Can you work these out from the model? Positions are in its coordinate system, mm. A direction names the side the tool comes from. Give positions to 0.01 mm unless a question says otherwise; leave off trailing zeros. Order: outer loops, then holes, each group sorted by start corner. A loop starts at its lowest first (then second) coordinate and runs counter-clockwise, first axis right, second up. Notation, with made-up numbers: (-36, 84) - (15, 84) arc R31 cw to (15, 118) - close; hole circle Ø8 at (-7.75, 62.25). An arc over 180 degrees is marked (long way). One line per question, with ' | ' between items.
```python
from build123d import *

# Parameters (mm, degrees)
ESQUISSE1_W             = 28.5
ESQUISSE1_H             = 46.6
BOSS_EXTRU_1_DEPTH      = 34
ESQUISSE2_R             = 10.15
BOSS_EXTRU_2_DEPTH      = 2
ESQUISSE3_R             = 1
ENL_V_MAT_EXTRU_1_DEPTH = 2


with BuildPart() as part:
    # Esquisse1 → Boss.-Extru.1 (new body)
    with BuildSketch(Plane.XY):
        Rectangle(ESQUISSE1_W, ESQUISSE1_H)
    extrude(amount=BOSS_EXTRU_1_DEPTH)

    # Esquisse2 → Boss.-Extru.2 (add)
    with BuildSketch(Plane.XY.offset(34)):
        with Locations((0, 12)):
            Circle(ESQUISSE2_R)
    extrude(amount=BOSS_EXTRU_2_DEPTH)

    # Esquisse3 → Enlèv. mat.-Extru.1 (cut)
    with BuildSketch(Plane(origin=(0, 23.3, 0), x_dir=(1, 0, 0), z_dir=(0, 1, 0))):
        with Locations(Location((-8.25, -25.319390083, 0), (0, 0, 270))):
            Circle(ESQUISSE3_R)
        with Locations(Location((8.25, -25.319390083, 0), (0, 0, 270))):
            Circle(ESQUISSE3_R)
    extrude(amount=-ENL_V_MAT_EXTRU_1_DEPTH, mode=Mode.SUBTRACT)


solid = part.part
```
(1) If I drill on line 1 (Z direction, x = -3, y = -17.5), over which ranges is the centre line in solid material (lowest first)?
Answer below:
line 1: 0 to 34
(2) On a 3-axis mill with a long thin cutter (end or side, diameter ignored), from which of +Z, -Z, +X, -X, +Y, -Y can I reach the whole of each face in a straight line? I mean faces 1 (the face through (8, 21.3, 25)), 2 (the face through (0, 0, 0)). Say none if no direction works.
Answer below:
face 1: +Y | face 2: -Z, +X, -X, +Y, -Y
(3) If we mould it in two halves opening along X, with no side actions, what happens to faces 3 (the face through (0, -5, 34)), 4 (the face through (-1.321, 22.064, 34.986)), 5 (the face through (14.25, 0, 17)), 6 (the face through (-7.574, 22.314, 24.582))? For each: released by +X, released by -X, zero draft, split by the parting line, or undercut.
Answer below:
face 3: zero draft | face 4: split by the parting line | face 5: released by +X | face 6: undercut
(4) Imagine slicing it at B-B (y = 4). List the corners of the cut face in (x, z) for me, and give its area (3 significant figures).
Answer below:
outline: (-14.25, 0) - (14.25, 0) - (14.25, 34) - (6.25, 34) - (6.25, 36) - (-6.25, 36) - (-6.25, 34) - (-14.25, 34) - close | area: 994 mm^2
(5) Imagine slicing it at C-C (x = -8.25). List the corners of the cut face in (y, z) for me.
Answer below:
outline: (-23.3, 0) - (23.3, 0) - (23.3, 24.32) - (21.3, 24.32) - (21.3, 26.32) - (23.3, 26.32) - (23.3, 34) - (17.91, 34) - (17.91, 36) - (6.09, 36) - (6.09, 34) - (-23.3, 34) - close
(6) Imagine slicing it at A-A (x = 0). List the corners of the cut face in (y, z) for me.
Answer below:
outline: (-23.3, 0) - (23.3, 0) - (23.3, 34) - (22.15, 34) - (22.15, 36) - (1.85, 36) - (1.85, 34) - (-23.3, 34) - close
(7) Will this pin go through, and if not, where does the flat tip stop? pin 1 (1.2 mm diameter, centred on x = 8.25, z = 25.32, fed in from +Y).
Answer below:
pin 1: y = 21.3
(8) Imagine slicing it at D-D (y = -16). List the corners of the cut face in (x, z) for me, and give its area (3 significant figures).
Answer below:
outline: (-14.25, 0) - (14.25, 0) - (14.25, 34) - (-14.25, 34) - close | area: 969 mm^2
